The model under review builds one solid part; all positions refer to its coordinate system, in mm. A direction names the side the tool comes from. Round coordinates to 2 decimals unless told otherwise and drop trailing zeros. Write each loop counter-clockwise with the first axis right and the second up, starting at its lowest first coordinate (ties: lowest second). Pieces come first, ordered by that corner, then holes. Notation, with made-up numbers: (42, 45.25) -> (97, 45.25) arc R17 cw to (97, 64.25) -> close; hole circle Ø5 at (-6.75, 32). An arc over 180 degrees is marked (long way). Answer as a JSON object with one key per item and string values. Group by question number.
1) We need section B-B, the plane y = -61. Write out the cut boundary in (x, z), then the cut area to 3 significant figures.
2) Machinability: for faces 5 (the flat face through (35, -56, 0)), 6 (the flat face through (6, -61, 1)), which of the approach directions +Z, -Z, +X, -X, +Y, -Y give a long, thin tool a straight path to every point of the face, cutting with its end or side? Answer none if there is none.
3) We need section D-D, the plane z = 1.9. Write out the cut boundary in (x, y), then the cut area to 3 significant figures.
4) We need section C-C, the plane x = 19. Write out the cut boundary in (y, z), then the cut area to 3 significant figures.
5) We need section A-A, the plane x = 38.5. Write out the cut boundary in (y, z), then the cut area to 3 significant figures.
6) Insertion check: pin 1 Ø2.5 at (x, y) = (38.5, -22) entering from +Z. The pin has a flat end and moves straight along its axis. Give the tip position at first contact, or say it passes through.
7) Mouldability with a two-part tool opening along Y and no side actions: class faces 1 (the flat face through (21, -8.003, 1)), 2 (the flat face through (34, -64, 2)), 3 (the flat face through (21, -106.003, 1)), 4 (the flat face through (35, -56, 3)) as pulls with the +Y half, pulls with the -Y half, needs draft (parallel to the pull), parting line crosses it, or undercut.
8) To check wall thickness, follow probe 1 along Y at (x, z) = (5.5, 1.45); probe 2 along Y at (x, z) = (12, 0.35); probe 3 along X at (y, z) = (-37, 2.6). State the ranges of each line that lie inside material, in increasing order. Write a range as [from, to].
from build123d import *

# Parameters (mm, degrees)
SKETCH1_W           = 30
SKETCH1_H           = 65
BOSS_EXTRUDE1_DEPTH = 3
SKETCH3_R           = 1
CUT_EXTRUDE1_DEPTH  = 3
SKETCH4_W           = 2
SKETCH4_H           = 65
BOSS_EXTRUDE2_DEPTH = 3


with BuildPart() as part:
    # Sketch1 → Boss-Extrude1 (new body)
    with BuildSketch(Plane.XY):
        Polygon((0, 0), (0, -114.006141835), (0, -92.003070917), (0, -106.003070917), (6, -106.003070917), (36, -106.003070917), (42, -106.003070917), (42, -92.003070917), (42, -114.006141835), (42, 0), (42, -22.003070917), (42, -8.003070917), (36, -8.003070917), (6, -8.003070917), (0, -8.003070917), (0, -22.003070917), align=None)
        with Locations((21, -63.503070917)):
            Rectangle(SKETCH1_W, SKETCH1_H, mode=Mode.SUBTRACT)
    extrude(amount=BOSS_EXTRUDE1_DEPTH)

    # Sketch3 → Cut-Extrude1 (cut)
    with BuildSketch(Plane(origin=(0, 0, 0), x_dir=(-1, 0, 0), z_dir=(0, 0, -1))):
        with Locations((-38.5, -22.003070917)):
            Circle(SKETCH3_R)
        with Locations((-5.5, -22.003070917)):
            Circle(SKETCH3_R)
        with Locations((-5.5, -92.003070917)):
            Circle(SKETCH3_R)
        with Locations((-38.5, -92.003070917)):
            Circle(SKETCH3_R)
    extrude(amount=-CUT_EXTRUDE1_DEPTH, mode=Mode.SUBTRACT)

    # Sketch4 → Boss-Extrude2 (add)
    with BuildSketch(Plane.XY.offset(3)):
        with Locations((35, -63.503070917)):
            Rectangle(SKETCH4_W, SKETCH4_H)
    extrude(amount=-BOSS_EXTRUDE2_DEPTH)


solid = part.part
Here are the results:
{
 "1": {"outline": "(0, 0) -> (6, 0) -> (6, 3) -> (0, 3) -> close; (34, 0) -> (42, 0) -> (42, 3) -> (34, 3) -> close", "area": "42.0 mm^2"},
 "2": {"face 5": "-Z, +X, -X, +Y, -Y", "face 6": "+Z, -Z"},
 "3": {"outline": "(0, -106) -> (42, -106) -> (42, -8) -> (0, -8) -> close; hole circle Ø2 at (5.5, -22); hole (6, -96) -> (34, -96) -> (34, -31) -> (6, -31) -> (6, -91.14) arc R1 ccw (long way) to (6, -92.87) -> close; hole circle Ø2 at (38.5, -92); hole circle Ø2 at (38.5, -22)", "area": "2,280 mm^2"},
 "4": {"outline": "(-106, 0) -> (-96, 0) -> (-96, 3) -> (-106, 3) -> close; (-31, 0) -> (-8, 0) -> (-8, 3) -> (-31, 3) -> close", "area": "99.0 mm^2"},
 "5": {"outline": "(-106, 0) -> (-93, 0) -> (-93, 3) -> (-106, 3) -> close; (-91, 0) -> (-23, 0) -> (-23, 3) -> (-91, 3) -> close; (-21, 0) -> (-8, 0) -> (-8, 3) -> (-21, 3) -> close", "area": "282 mm^2"},
 "6": {"pin 1": "stops at z = 3"},
 "7": {"face 1": "pulls with the +Y half", "face 2": "undercut", "face 3": "pulls with the -Y half", "face 4": "needs draft"},
 "8": {"probe 1": "y = [-106, -93], [-91, -23], [-21, -8]", "probe 2": "y = [-106, -96], [-31, -8]", "probe 3": "x = [0, 6], [34, 42]"}
}
